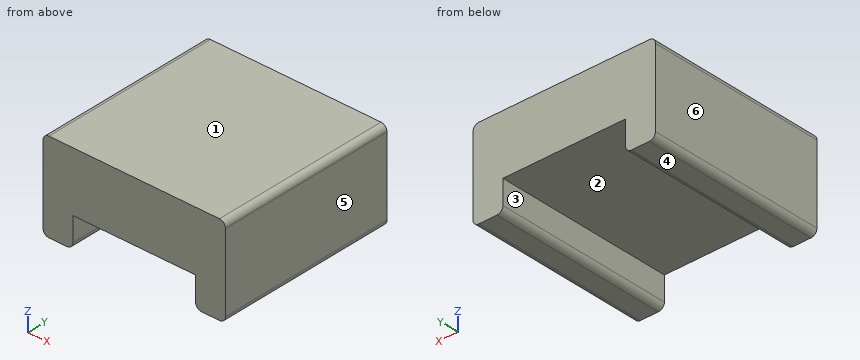
Autodesk Fusion 360 part; units mm, degrees
sketch "Sketch1" plane through (0, 0, 0) normal (0, 0, 1) x (1, 0, 0)
  line L0 (10.25, 15) -> (-10.25, 15)
  line L1 (-10.25, 15) -> (-10.25, -15)
  line L2 (-10.25, -15) -> (10.25, -15)
  line L3 (10.25, -15) -> (10.25, 15)
  line L4 (10.25, 15) -> (-10.25, -15) construction
  line L5 (-10.25, 15) -> (10.25, -15) construction
  line L6 (-10.25, 15) -> (-15.25, 15)
  line L7 (-15.25, 15) -> (-15.25, -15)
  line L8 (-15.25, -15) -> (-10.25, -15)
  line L9 (-10.25, -15) -> (-10.25, 15)
  line L10 (10.25, 15) -> (15.25, 15)
  line L11 (15.25, 15) -> (15.25, -15)
  line L12 (15.25, -15) -> (10.25, -15)
  line L13 (10.25, -15) -> (10.25, 15)
  dimension "d1" = 20.5
  dimension "d2" = 30
  dimension "d3" = 5
  dimension "d4" = 30
  dimension "d5" = 5
  dimension "d6" = 30
extrude "Extrude1" add sketch "Sketch1" along normal blind 10
extrude "Extrude2" add sketch "Sketch1" against normal blind 5 contours L3 L10 L11 L12 L13 | L1 L6 L7 L8 L9
fillet "Fillet1" radius 1 6 edges at (-10.25, 0, -5) (10.25, 0, -5) (15.25, 0, -5) (-15.25, 0, -5) (-15.25, 0, 10) (15.25, 0, 10)
Model file for the job. Use its own axes, mm. Face numbers are marked on the shaded views. A direction names the side the tool comes from. Give positions to 0.01 mm unless a question says otherwise; leave off trailing zeros. Loops run counter-clockwise (first coordinate to the right, second up) from the corner with the lowest first, then second, coordinate; pieces in that order, holes last.
Item 1: Slice it at B-B (x = 0). Write the cut outline in (y, z).
Check values:
outline: (-15, 0) - (15, 0) - (15, 10) - (-15, 10) - close
Item 2: Mould opens along X. For the marked faces 3, 4, 5 and 6 say: +X half, -X half, draft (parallel to the pull), parting line (faces both ways), or undercut.
Check values:
face 3: undercut
face 4: draft
face 5: +X half
face 6: -X half
Item 3: Which spindle directions (+Z, -Z, +X, -X, +Y, -Y) get a long thin tool onto all of the face, cutting with end or side? Do the marked faces 1 and 2. Say none if no direction does.
Check values:
face 1: +Z, +X, -X, +Y, -Y
face 2: -Z, +Y, -Y
Item 4: Slice it at A-A (y = 5). Write the cut outline in (x, z).
Check values:
outline: (-15.25, -4) arc R1 ccw to (-14.25, -5) - (-11.25, -5) arc R1 ccw to (-10.25, -4) - (-10.25, 0) - (10.25, 0) - (10.25, -4) arc R1 ccw to (11.25, -5) - (14.25, -5) arc R1 ccw to (15.25, -4) - (15.25, 9) arc R1 ccw to (14.25, 10) - (-14.25, 10) arc R1 ccw to (-15.25, 9) - close
Item 5: Drop flat-ended pins along their axis: P1, Ø1.5, axis at x = -4.5, z = -1, coming from the -Y side; P2, Ø8, axis at x = -8, y = 12, coming from the -Z side. Give the stop position or say it passes through.
Check values:
P1: passes through
P2: stops at z = -5
Item 6: Drill centre lines: line 1 along X through (y, z) = (9.75, -3.75); line 2 along Z through (x, y) = (-3, -8.5). Where is each one in solid material? Low to high.
Check values:
line 1: x = -15.25 to -10.25, 10.25 to 15.25
line 2: z = 0 to 10
